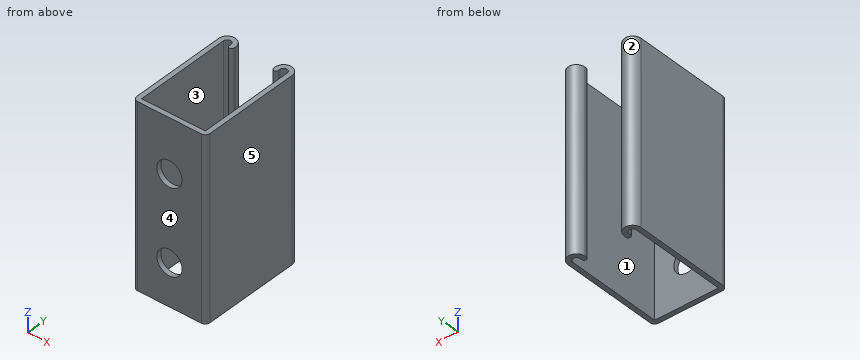
from build123d import *

# Parameters (mm, degrees)
BASE_EXTRUDE_DEPTH = 101.6
HOLE1_START        = -28.0162
HOLE1_OUTLINE_R    = 7.14375
HOLE1_DEPTH        = 2.6924
LPATTERN2_COUNT    = 2
LPATTERN2_PITCH    = 47.625


# Read off the part's stored shape, not the designer's step: Hole1
with BuildPart() as part:
    # Sketch1 → Base-Extrude (new body)
    with BuildSketch(Plane.XY):
        with BuildLine():
            Line((-20.6375, 29.1719), (-20.6375, -25.3238))
            ThreePointArc((-20.6375, -25.3238), (-19.848914298, -27.227614298), (-17.9451, -28.0162))
            Line((-17.9451, -28.0162), (17.9451, -28.0162))
            ThreePointArc((17.9451, -28.0162), (19.848914298, -27.227614298), (20.6375, -25.3238))
            Line((20.6375, -25.3238), (20.6375, 29.1719))
            ThreePointArc((20.6375, 29.1719), (15.875, 33.9344), (11.1125, 29.1719))
            Line((11.1125, 29.1719), (11.1125, 28.13685))
            ThreePointArc((11.1125, 28.13685), (12.4587, 26.79065), (13.8049, 28.13685))
            Line((13.8049, 28.13685), (13.8049, 29.1719))
            ThreePointArc((13.8049, 29.1719), (15.875, 31.242), (17.9451, 29.1719))
            Line((17.9451, 29.1719), (17.9451, -25.3238))
            Line((17.9451, -25.3238), (-17.9451, -25.3238))
            Line((-17.9451, -25.3238), (-17.9451, 29.1719))
            ThreePointArc((-17.9451, 29.1719), (-15.875, 31.242), (-13.8049, 29.1719))
            Line((-13.8049, 29.1719), (-13.8049, 28.13685))
            ThreePointArc((-13.8049, 28.13685), (-12.4587, 26.79065), (-11.1125, 28.13685))
            Line((-11.1125, 28.13685), (-11.1125, 29.1719))
            ThreePointArc((-11.1125, 29.1719), (-15.875, 33.9344), (-20.6375, 29.1719))
        make_face()
    extrude(amount=BASE_EXTRUDE_DEPTH)

    # Hole1 outline → Hole1 (cut)
    with BuildSketch(Plane(origin=(0, 0, 0), x_dir=(1, 0, 0), z_dir=(0, 1, 0)).offset(HOLE1_START)):
        with Locations((0, -23.8125)):
            Circle(HOLE1_OUTLINE_R)
    hole1 = extrude(amount=HOLE1_DEPTH, mode=Mode.SUBTRACT)

    # LPattern2: Hole1 ×2
    with Locations(*[(0, 0, i * LPATTERN2_PITCH) for i in range(1, LPATTERN2_COUNT)]):
        add(hole1, mode=Mode.SUBTRACT)


solid = part.part
The listing builds one solid part. Answer for the finished solid, in the listing's coordinates (mm). Face numbers are marked on the shaded views. A direction names the side the tool comes from. Round coordinates to 2 decimals unless told otherwise and drop trailing zeros. Write each loop counter-clockwise with the first axis right and the second up, starting at its lowest first coordinate (ties: lowest second). Pieces come first, ordered by that corner, then holes. Notation, with made-up numbers: M 4.25,-12.5 L 61.25,-12.5 A20 ccw 61.25,6.5 Z; hole C -27,79.25 d10. An arc over 180 degrees is marked long. Write each question's results on one line, items separated by ' | '. Start each with the question number.
Item 1: For the marked faces 1 and 2, determine the directions among +Z, -Z, +X, -X, +Y, -Y from which every point of the face is accessible in a straight line to the end or side of a thin tool.
Item 2: A cutting plane is placed at A-A on x = 0. Write down the section's boundary in (y, z).
Item 3: Flat-ended cylindrical pins translate along their axes: pin 1 Ø11.5 at (x, z) = (0, 71.44) entering from -Y; pin 2 Ø18 at (x, z) = (6, 49.5) entering from +Y; pin 3 Ø3 at (x, z) = (-8, 17.5) entering from +Y. Find the tip coordinate at first contact, or state that the pin passes through.
Item 4: A cutting plane is placed at C-C on z = 73. Write down the section's boundary in (x, y) (1 decimal).
Item 5: Straight lines are drawn through the part: L1, parallel to Z at x = 0, y = -27.2; L2, parallel to X at y = 24.5, z = 42; L3, parallel to Y at x = 10, z = 54. For each, find the intervals that lie inside material, in ascending order. Write a range as [from, to].
Item 6: For a pull along X with two mould halves and no side action, classify the marked faces 3, 4 and 5 as pulls with the +X half, pulls with the -X half, needs draft (parallel to the pull), parting line crosses it, or undercut.
Item 7: A cutting plane is placed at B-B on y = -12.5. Write down the section's boundary in (x, z), and give its area (3 significant figures).
Item 8: A cutting plane is placed at D-D on z = 35.5. Write down the section's boundary in (x, y) (1 decimal), and give its area (3 significant figures).
Check sheet entries:
1) face 1: +Z, -Z | face 2: +Z, -Z, +Y
2) outline: M -28.02,0 L -25.32,0 L -25.32,16.67 L -28.02,16.67 Z; M -28.02,30.96 L -25.32,30.96 L -25.32,64.29 L -28.02,64.29 Z; M -28.02,78.58 L -25.32,78.58 L -25.32,101.6 L -28.02,101.6 Z
3) pin 1: through | pin 2: y = 33.85 | pin 3: y = -25.32
4) outline: M -20.6,-25.3 A2.7 ccw -17.9,-28 L -7,-28 L -7,-25.3 L -17.9,-25.3 L -17.9,29.2 A2.1 cw -13.8,29.2 L -13.8,28.1 A1.3 ccw -11.1,28.1 L -11.1,29.2 A4.8 ccw -20.6,29.2 Z; M 7,-28 L 17.9,-28 A2.7 ccw 20.6,-25.3 L 20.6,29.2 A4.8 ccw 11.1,29.2 L 11.1,28.1 A1.3 ccw 13.8,28.1 L 13.8,29.2 A2.1 cw 17.9,29.2 L 17.9,-25.3 L 7,-25.3 Z
5) L1: [0, 16.67], [30.96, 64.29], [78.58, 101.6] | L2: [-20.64, -17.95], [17.95, 20.64] | L3: [-28.02, -25.32]
6) face 3: undercut | face 4: needs draft | face 5: pulls with the +X half
7) outline: M -20.64,0 L -17.95,0 L -17.95,101.6 L -20.64,101.6 Z; M 17.95,0 L 20.64,0 L 20.64,101.6 L 17.95,101.6 Z | area: 547 mm²
8) outline: M -20.6,-25.3 A2.7 ccw -17.9,-28 L 17.9,-28 A2.7 ccw 20.6,-25.3 L 20.6,29.2 A4.8 ccw 11.1,29.2 L 11.1,28.1 A1.3 ccw 13.8,28.1 L 13.8,29.2 A2.1 cw 17.9,29.2 L 17.9,-25.3 L -17.9,-25.3 L -17.9,29.2 A2.1 cw -13.8,29.2 L -13.8,28.1 A1.3 ccw -11.1,28.1 L -11.1,29.2 A4.8 ccw -20.6,29.2 Z | area: 471 mm²
